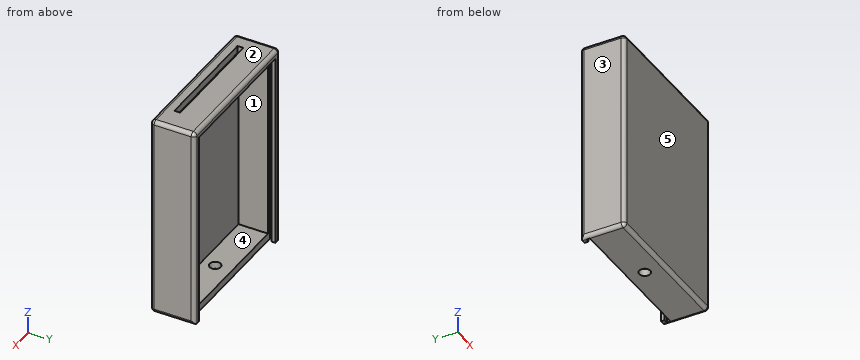
Autodesk Inventor part; units mm, degrees
ref_plane "YZ Plane" through (0, 0, 0) normal (1, 0, 0) x (0, 1, 0)
ref_plane "XZ Plane" through (0, 0, 0) normal (0, 1, 0) x (-1, 0, 0)
ref_plane "XY Plane" through (0, 0, 0) normal (0, 0, 1) x (1, 0, 0)
sketch "スケッチ1" plane through (0, 0, 0) normal (0, 1, 0) x (-1, 0, 0)
  line L0 (0, 0) -> (-41, 0)
  line L1 (-41, 0) -> (-41, -55)
  line L2 (-41, -55) -> (0, -55)
  line L3 (0, -55) -> (0, 0)
  dimension "d0" = 41
  dimension "d1" = 55
extrude "押し出し1" add sketch "スケッチ1" along normal blind 12
sketch "スケッチ3" plane through (0, 12, 0) normal (0, 1, 0) x (1, 0, 0)
  line L0 (2, 2) -> (39, 2)
  line L1 (39, 2) -> (39, 53)
  line L2 (39, 53) -> (2, 53)
  line L3 (2, 53) -> (2, 2)
  line L4 (0, 55) -> (0, 0)
  line L5 (0, 0) -> (41, 0)
  dimension "d4" = 37
  dimension "d5" = 51
  dimension "d6" = 2
  dimension "d7" = 2
extrude "押し出し2" cut sketch "スケッチ3" against normal blind 10
sketch "スケッチ4" plane through (0, 0, 0) normal (0, 0, 1) x (1, 0, 0)
  line L0 (4.25, 4.6) -> (34.75, 4.6)
  line L1 (34.75, 4.6) -> (34.75, 3)
  line L2 (34.75, 3) -> (4.25, 3)
  line L3 (4.25, 3) -> (4.25, 4.6)
  line L4 (0, 0) -> (41, 0)
  line L5 (0, 0) -> (0, 12)
  point P0 (4.25, 3.8)
  point P1 (19.5, 4.6)
  dimension "d10" = 30.5
  dimension "d11" = 1.6
  dimension "d12" = 3
  dimension "d14" = 19.5
extrude "押し出し3" cut sketch "スケッチ4" against normal blind 10
sketch "スケッチ5" plane through (41, 0, -55) normal (0, 0, -1) x (-1, 0, 0)
  circle A0 centre (21.5, 5.5) radius 1.5
  line L0 (41, 0) -> (41, 12)
  line L1 (0, 12) -> (41, 12)
  dimension "d17" = 3
  dimension "d18" = 19.5
  dimension "d19" = 6.5
extrude "押し出し4" cut sketch "スケッチ5" against normal blind 10
sketch "スケッチ7" plane through (41, 0, -55) normal (0, 0, -1) x (-1, 0, 0)
  line L0 (40, 11) -> (1, 11)
  line L1 (1, 11) -> (1, 10)
  line L2 (1, 10) -> (40, 10)
  line L3 (40, 10) -> (40, 11)
  line L4 (41, 0) -> (41, 12)
  line L5 (0, 12) -> (41, 12)
  point P0 (20.5, 10)
  dimension "d22" = 39
  dimension "d23" = 1
  dimension "d24" = 20.5
  dimension "d25" = 1
extrude "押し出し5" cut sketch "スケッチ7" against normal blind 54
sketch "スケッチ8" plane through (41, 0, -55) normal (0, 0, -1) x (-1, 0, 0)
  line L0 (39, 12) -> (2, 12)
  line L1 (2, 12) -> (2, 11)
  line L2 (2, 11) -> (39, 11)
  line L3 (39, 11) -> (39, 12)
  line L4 (41, 0) -> (41, 12)
  line L5 (0, 12) -> (41, 12)
  point P0 (20.5, 12)
  dimension "d28" = 37
  dimension "d29" = 1
  dimension "d30" = 20.5
  dimension "d31" = 0
extrude "押し出し6" cut sketch "スケッチ8" against normal blind 2
fillet "フィレット1" radius 1 11 edges at (0, 6, 0) (41, 6, 0) (20.5, 12, 0) (41, 12, -27.5) (20.5, 0, -55) (0, 6, -55) (0, 0, -27.5) (20.5, 0, 0) (41, 0, -27.5) (41, 6, -55) (0, 12, -27.5)
properties part number "case_basic"
Geometry check sheet. Reference: the model listing, model coordinates, mm. Face numbers are marked on the shaded views. A direction names the side the tool comes from. Give positions to 0.01 mm unless a question says otherwise; leave off trailing zeros. Loops run counter-clockwise (first coordinate to the right, second up) from the corner with the lowest first, then second, coordinate; pieces in that order, holes last. Notation, with made-up numbers: M -34,-5.75 L -2,-5.75 A15 ccw -2,11.25 Z; hole C -2,19 d5. An arc over 180 degrees is marked long. Answer as a JSON object with one key per item and string values. Group by question number.
Item 1: Sectioned sample at A-A on y = 8.25. Record the boundary of the cut face in (x, z).
Item 2: Sectioned sample at B-B on x = 30. Record the boundary of the cut face in (y, z), plus the area to 3 significant figures.
Item 3: Gauge pin test, flat ends, axial feed: pin 1 (0.5 mm diameter, centred on x = 15.5, y = 10.5, fed in from -Z); pin 2 (0.8 mm diameter, centred on x = 17, y = 11.5, fed in from -Z); pin 3 (6 mm diameter, centred on x = 28.5, z = -49, fed in from +Y). Record the tip position at first contact, or that the pin passes through.
Item 4: Material ranges on L1, parallel to Y at x = 19.5, z = -53.5; L2, parallel to Z at x = 3, y = 5; L3, parallel to Z at x = 6.5, y = 10.75, recorded low to high.
Item 5: Mould release check, pull along X, two halves, no side actions. Record for the marked faces 3, 4 and 5: pulls with the +X half, pulls with the -X half, needs draft (parallel to the pull), parting line crosses it, or undercut.
Item 6: Access from +Z, -Z, +X, -X, +Y, -Y to the whole of each face (thin tool, end or side, straight path). Record for the marked faces 1 and 2.
Item 7: Sectioned sample at D-D on x = 19.5. Record the boundary of the cut face in (y, z).
Item 8: Sectioned sample at C-C on z = -36. Record the boundary of the cut face in (x, y).
Findings below:
{
 "1": {"outline": "M 0,-54 A1 ccw 1,-55 L 40,-55 A1 ccw 41,-54 L 41,-1 A1 ccw 40,0 L 1,0 A1 ccw 0,-1 Z; hole M 2,-53 L 39,-53 L 39,-2 L 2,-2 Z"},
 "2": {"outline": "M 0,-54 A1 ccw 1,-55 L 10,-55 L 10,-53 L 2,-53 L 2,-2 L 3,-2 L 3,0 L 1,0 A1 ccw 0,-1 Z; M 4.6,-2 L 10,-2 L 10,-1 L 11,-1 L 11,-2 L 12,-2 L 12,-1 A1 ccw 11,0 L 4.6,0 Z", "area": "141 mm2"},
 "3": {"pin 1": "z = -1", "pin 2": "z = -2", "pin 3": "y = 2"},
 "4": {"L1": "0 to 4, 7 to 10", "L2": "-55 to -53, -2 to 0", "L3": "-1 to 0"},
 "5": {"face 3": "pulls with the -X half", "face 4": "undercut", "face 5": "needs draft"},
 "6": {"face 1": "+Y", "face 2": "+Z, +X, -X, +Y, -Y"},
 "7": {"outline": "M 0,-54 A1 ccw 1,-55 L 4,-55 L 4,-53 L 2,-53 L 2,-2 L 3,-2 L 3,0 L 1,0 A1 ccw 0,-1 Z; M 4.6,-2 L 10,-2 L 10,-1 L 11,-1 L 11,-2 L 12,-2 L 12,-1 A1 ccw 11,0 L 4.6,0 Z; M 7,-55 L 10,-55 L 10,-53 L 7,-53 Z"},
 "8": {"outline": "M 0,1 A1 ccw 1,0 L 40,0 A1 ccw 41,1 L 41,11 A1 ccw 40,12 L 39,12 L 39,11 L 40,11 L 40,10 L 39,10 L 39,2 L 2,2 L 2,10 L 1,10 L 1,11 L 2,11 L 2,12 L 1,12 A1 ccw 0,11 Z"}
}
